Geometry check sheet. Reference: the model listing, model coordinates, mm. A direction names the side the tool comes from. Coordinates: 2 decimals unless noted, no trailing zeros. Write each loop counter-clockwise with the first axis right and the second up, starting at its lowest first coordinate (ties: lowest second). Pieces come first, ordered by that corner, then holes. Notation, with made-up numbers: (84, 8.5) -> (123, 8.5) arc R28 cw to (123, 27.5) -> close; hole circle Ø9 at (6.5, -30.5). An arc over 180 degrees is marked (long way). Use a Markdown table: item, result.
```python
from build123d import *

# Parameters (mm, degrees)
SKETCH2_R           = 63.5
BOSS_EXTRUDE1_DEPTH = 15.24
CUT_EXTRUDE3_DEPTH  = 92.086539071
SKETCH4_R           = 1.75
CUT_EXTRUDE4_DEPTH  = 55.626
SKETCH5_R           = 12.5
CUT_EXTRUDE5_DEPTH  = 5.334


with BuildPart() as part:
    # Sketch2 → Boss-Extrude1 (new body)
    with BuildSketch(Plane(origin=(0, 0, 0), x_dir=(1, 0, 0), z_dir=(0, 1, 0))):
        with Locations(Location((0, 0, 0), (0, 0, 90))):
            Circle(SKETCH2_R)
    extrude(amount=BOSS_EXTRUDE1_DEPTH)

    # Sketch3 → Cut-Extrude3 (cut, through all)
    with BuildSketch(Plane(origin=(0, 15.24, 0), x_dir=(1, 0, 0), z_dir=(0, 1, 0))):
        with BuildLine():
            ThreePointArc((2.683094535, 0), (-2.104641397, 1.664175734), (0.618701471, -2.610786237))
            Line((0.618701471, -2.610786237), (2.670795382, -0.25660926))
            ThreePointArc((2.670795382, -0.25660926), (2.680017983, -0.128451918), (2.683094535, 0))
        make_face()
    extrude(amount=-CUT_EXTRUDE3_DEPTH, mode=Mode.SUBTRACT)

    # Sketch4 → Cut-Extrude4 (cut)
    with BuildSketch(Plane(origin=(0, 15.24, 0), x_dir=(1, 0, 0), z_dir=(0, 1, 0))):
        with Locations(Location((-15.5, 15.5, 0), (0, 0, 270))):
            Circle(SKETCH4_R)
        with Locations(Location((15.5, 15.5, 0), (0, 0, 270))):
            Circle(SKETCH4_R)
        with Locations(Location((15.5, -15.5, 0), (0, 0, 270))):
            Circle(SKETCH4_R)
        with Locations(Location((-15.5, -15.5, 0), (0, 0, 270))):
            Circle(SKETCH4_R)
    extrude(amount=-CUT_EXTRUDE4_DEPTH, mode=Mode.SUBTRACT)

    # Sketch5 → Cut-Extrude5 (cut)
    with BuildSketch(Plane(origin=(0, 15.24, 0), x_dir=(1, 0, 0), z_dir=(0, 1, 0))):
        with Locations(Location((0, 0, 0), (0, 0, 270))):
            Circle(SKETCH5_R)
    extrude(amount=-CUT_EXTRUDE5_DEPTH, mode=Mode.SUBTRACT)


solid = part.part
```
Item 1: Depth check by flat-ended pin: P1, Ø2, axis at x = -19, y = 4, coming from the +Z side; P2, Ø5, axis at y = 5, z = 21.5, coming from the +X side; P3, Ø3, axis at x = -14.5, y = 8.5, coming from the +Z side. Enter the tip coordinate at first touch or a pass-through.
Answer block:
| item | result |
|---|---|
| P1 | stops at z = 60.9 |
| P2 | stops at x = 60.59 |
| P3 | stops at z = 62.16 |
Item 2: Thickness scan on L1, parallel to X at y = 12.55, z = 0; L2, parallel to Z at x = -15, y = 0.5; L3, parallel to Z at x = 14, y = 5.25. Record the ranges inside material, lowest first. Write a range as [from, to].
Answer block:
| item | result |
|---|---|
| L1 | x = [-63.5, -12.5], [12.5, 63.5] |
| L2 | z = [-61.7, -17.18], [-13.82, 13.82], [17.18, 61.7] |
| L3 | z = [-61.94, -16.4], [-14.6, 14.6], [16.4, 61.94] |
Item 3: Section check C-C on x = -15.5. Record the boundary of the cut face in (y, z), then the cut area to 3 significant figures.
Answer block:
| item | result |
|---|---|
| outline | (0, -61.58) -> (15.24, -61.58) -> (15.24, -17.25) -> (0, -17.25) -> close; (0, -13.75) -> (15.24, -13.75) -> (15.24, 13.75) -> (0, 13.75) -> close; (0, 17.25) -> (15.24, 17.25) -> (15.24, 61.58) -> (0, 61.58) -> close |
| area | 1,770 mm^2 |
Item 4: Mould release check, pull along X, two halves, no side actions. Record for faces 1 (the cylindrical face through (61.99, 7.51, 13.77)), 2 (the flat face through (13, 15.24, 1)), 3 (the cylindrical face through (17.235, 7.727, 15.272)): +X half, -X half, draft (parallel to the pull), parting line (faces both ways), or undercut.
Answer block:
| item | result |
|---|---|
| face 1 | parting line |
| face 2 | draft |
| face 3 | undercut |
Item 5: Section check D-D on x = 5. Record the boundary of the cut face in (y, z).
Answer block:
| item | result |
|---|---|
| outline | (0, -63.3) -> (15.24, -63.3) -> (15.24, -11.46) -> (9.91, -11.46) -> (9.91, 11.46) -> (15.24, 11.46) -> (15.24, 63.3) -> (0, 63.3) -> close |
Item 6: Section check B-B on z = 15.5. Record the boundary of the cut face in (x, y), then the cut area to 3 significant figures.
Answer block:
| item | result |
|---|---|
| outline | (-61.58, 0) -> (-17.25, 0) -> (-17.25, 15.24) -> (-61.58, 15.24) -> close; (-13.75, 0) -> (13.75, 0) -> (13.75, 15.24) -> (-13.75, 15.24) -> close; (17.25, 0) -> (61.58, 0) -> (61.58, 15.24) -> (17.25, 15.24) -> close |
| area | 1,770 mm^2 |
Item 7: Section check A-A on y = 2.75. Record the boundary of the cut face in (x, z).
Answer block:
| item | result |
|---|---|
| outline | circle Ø127 at (0, 0); hole circle Ø3.5 at (-15.5, -15.5); hole circle Ø3.5 at (-15.5, 15.5); hole (0.62, 2.61) arc R2.68 ccw (long way) to (2.67, 0.26) -> close; hole circle Ø3.5 at (15.5, -15.5); hole circle Ø3.5 at (15.5, 15.5) |
Item 8: Tool access check on faces 4 (the cylindrical face through (3.755, 12.61, 11.923)), 5 (the cylindrical face through (-13.765, 7.727, 15.272)). Record the directions out of +Z, -Z, +X, -X, +Y, -Y that give a thin tool (end or side, any length) a straight path to the whole face; none if there is none.
Answer block:
| item | result |
|---|---|
| face 4 | +Y |
| face 5 | +Y, -Y |
